```python
from build123d import *

# Parameters (mm, degrees)
SKETCH1_R           = 1.524
BOSS_EXTRUDE1_DEPTH = 4.7625
SKETCH2_R           = 1.1303
CUT_EXTRUDE1_DEPTH  = 6.35
CUT_EXTRUDE2_START  = -6.35
SKETCH3_R           = 1.1303
CUT_EXTRUDE2_DEPTH  = 6.35


with BuildPart() as part:
    # Sketch1 → Boss-Extrude1 (new body)
    with BuildSketch(Plane.XY):
        Polygon((-46.0375, 0), (46.0375, 0), (46.0375, 10.16), (41.275, 10.16), (41.275, 20.32), (-41.275, 20.32), (-41.275, 10.16), (-46.0375, 10.16), align=None)
        with Locations(Location((-43.65625, 5.08, 0), (0, 0, 180))):
            Circle(SKETCH1_R, mode=Mode.SUBTRACT)
        with Locations(Location((43.65625, 5.08, 0), (0, 0, 180))):
            Circle(SKETCH1_R, mode=Mode.SUBTRACT)
    extrude(amount=BOSS_EXTRUDE1_DEPTH)

    # Sketch2 → Cut-Extrude1 (cut)
    with BuildSketch(Plane(origin=(41.275, 0, 0), x_dir=(0, 0, -1), z_dir=(1, 0, 0))):
        with Locations(Location((-2.38125, 15.24, 0), (0, 0, 90))):
            Circle(SKETCH2_R)
    extrude(amount=-CUT_EXTRUDE1_DEPTH, mode=Mode.SUBTRACT)

    # Sketch3 → Cut-Extrude2 (cut)
    with BuildSketch(Plane.ZY.offset(41.275).offset(CUT_EXTRUDE2_START)):
        with Locations(Location((2.38125, 15.24, 0), (0, 0, 90))):
            Circle(SKETCH3_R)
    extrude(amount=CUT_EXTRUDE2_DEPTH, mode=Mode.SUBTRACT)


solid = part.part
```
Geometry: final body of the model. Coordinates: model frame, mm. A direction names the side the tool comes from. Round coordinates to 2 decimals unless told otherwise and drop trailing zeros. Write each loop counter-clockwise with the first axis right and the second up, starting at its lowest first coordinate (ties: lowest second). Pieces come first, ordered by that corner, then holes.
Item 1: Mould query, pull axis Z, two halves, no side actions, for faces 4 (the face through (-41.275, 16.44, 2.88)), 5 (the face through (-1, 10, 4.762)), 6 (the face through (34.925, 15, 2)). Classes: +Z half, -Z half, draft (parallel to the pull), parting line (faces both ways), or undercut.
Item 2: Pin query (flat end, axial travel): P1, Ø1.8, axis at x = -43.66, y = 5.08, coming from the -Z side; P2, Ø1.4, axis at y = 14, z = 3, coming from the -X side (3 decimals); P3, Ø1.4, axis at y = 16, z = 2.5, coming from the +X side (3 decimals); P4, Ø2.5, axis at x = 44.5, z = 3, coming from the +Y side. Return the tip coordinate at first contact, or that it passes through.
Item 3: Material intervals for L1, parallel to X at y = 5.08, z = 1.4; L2, parallel to Z at x = -38, y = 15.24; L3, parallel to X at y = 3.75, z = 3.45, sorted ascending.
Item 4: Section query A-A (y = 15.24). Return loops of the section in (x, z) (1 decimal).
Item 5: Section query B-B (y = 5.08). Return loops of the section in (x, z).
Item 6: Section query C-C (x = -38). Return loops of the section in (y, z), plus the area to 3 significant figures.
Item 7: Set-up query: faces 1 (the face through (38.144, 16.284, 1.948)), 2 (the face through (44, 10.16, 2)), 3 (the face through (-38.056, 16.284, 2.814)). Return all of +Z, -Z, +X, -X, +Y, -Y with unobstructed straight access to the full face (end or side cutting, diameter ignored); none if empty.
Completed:
1. face 4: draft
1. face 5: +Z half
1. face 6: undercut
2. P1: passes through
2. P2: stops at x = -41.275
2. P3: stops at x = 41.275
2. P4: stops at y = 10.16
3. L1: x = -46.04 to -45.18, -42.13 to 42.13, 45.18 to 46.04
3. L2: z = 0 to 1.25, 3.51 to 4.76
3. L3: x = -46.04 to -44.4, -42.91 to 42.91, 44.4 to 46.04
4. outline: (-41.3, 0) - (41.3, 0) - (41.3, 1.3) - (34.9, 1.3) - (34.9, 3.5) - (41.3, 3.5) - (41.3, 4.8) - (-41.3, 4.8) - (-41.3, 3.5) - (-34.9, 3.5) - (-34.9, 1.3) - (-41.3, 1.3) - close
5. outline: (-46.04, 0) - (-45.18, 0) - (-45.18, 4.76) - (-46.04, 4.76) - close; (-42.13, 0) - (42.13, 0) - (42.13, 4.76) - (-42.13, 4.76) - close; (45.18, 0) - (46.04, 0) - (46.04, 4.76) - (45.18, 4.76) - close
6. outline: (0, 0) - (20.32, 0) - (20.32, 4.76) - (0, 4.76) - close; hole circle Ø2.26 at (15.24, 2.38)
6. area: 92.8 mm2
7. face 1: +X
7. face 2: +Z, -Z, +X, +Y
7. face 3: -X
